Autodesk Inventor part; units mm, degrees
ref_plane "YZ Plane" through (0, 0, 0) normal (1, 0, 0) x (0, 1, 0)
ref_plane "XZ Plane" through (0, 0, 0) normal (0, 1, 0) x (-1, 0, 0)
ref_plane "XY Plane" through (0, 0, 0) normal (0, 0, 1) x (1, 0, 0)
sketch "Sketch1" plane through (0, 0, 0) normal (0, 1, 0) x (-1, 0, 0)
  line L0 (19, 32.5) -> (-11, 32.5)
  line L1 (-11, -32.5) -> (19, -32.5)
  line L2 (19, -32.5) -> (19, 32.5)
  line L3 (19, 32.5) -> (-19, -32.5) construction
  line L4 (-19, 32.5) -> (19, -32.5) construction
  line L5 (19, 19) -> (-19, 19) construction
  line L6 (-19, 19) -> (-19, -19) construction
  line L7 (-19, -19) -> (19, -19) construction
  line L8 (19, -19) -> (19, 19) construction
  line L9 (19, 19) -> (-19, -19) construction
  line L10 (-19, 19) -> (19, -19) construction
  line L11 (19, 32.5) -> (-11, 32.5) construction
  line L12 (-11, 32.5) -> (-11, -32.5) construction
  line L13 (-11, -32.5) -> (19, -32.5) construction
  line L14 (19, -32.5) -> (19, 32.5) construction
  line L15 (-21.9768, -11.3147) -> (-19, 12.5) construction
  line L16 (15.5, 29) -> (-7.5, 29) construction
  line L17 (-7.5, 29) -> (-7.5, -29) construction
  line L18 (-7.5, -29) -> (15.5, -29) construction
  line L19 (15.5, -29) -> (15.5, 29) construction
  line L20 (15, 15) -> (-15, 15) construction
  line L21 (-15, 15) -> (-15, -15) construction
  line L22 (-15, -15) -> (15, -15) construction
  line L23 (15, -15) -> (15, 15) construction
  line L24 (15, 15) -> (-15, -15) construction
  line L25 (-15, 15) -> (15, -15) construction
  circle A0 centre (15, 15) radius 1.25
  circle A1 centre (15, -15) radius 1.25
  circle A2 centre (-15, -15) radius 1.25
  circle A3 centre (-15, 15) radius 1.25
  circle A4 centre (-7.5, 29) radius 1.25
  circle A5 centre (15.5, 29) radius 1.25
  circle A6 centre (15.5, -29) radius 1.25
  circle A7 centre (-7.5, -29) radius 1.25
  circle A8 centre (0, 12) radius 2.5 construction
  circle A9 centre (0, -12) radius 2.5 construction
  line L26 (-4.75, 25.5) -> (-10.25, 25.5)
  line L27 (-10.25, 25.5) -> (-10.25, -25.5) construction
  line L28 (-10.25, -25.5) -> (-4.75, -25.5)
  line L29 (-4.75, -25.5) -> (-4.75, 25.5) construction
  line L30 (-4.75, 25.5) -> (-10.25, -25.5) construction
  line L31 (-10.25, 25.5) -> (-4.75, -25.5) construction
  line L32 (-11, 32.5) -> (-19, 32.5)
  line L33 (-19, 32.5) -> (-19, 19)
  line L34 (-19, -19) -> (-19, -32.5)
  line L35 (-19, -32.5) -> (-11, -32.5)
  arc A10 (-14.9077, -17.4983) -> (-15, -12.5) centre (-15, -15) ccw
  arc A11 (-15, 12.5) -> (-14.9077, 17.4983) centre (-15, 15) ccw
  line L36 (-15, 12.5) -> (-19, 12.5)
  line L37 (-19, 12.5) -> (-19, 19)
  line L38 (-15, -12.5) -> (-19, -12.5)
  line L39 (-19, -12.5) -> (-19, -19)
  line L40 (-14.9077, -17.4983) -> (-14.9077, -19)
  line L41 (-14.9077, 17.4983) -> (-14.9077, 19)
  arc A12 (15, 17.5) -> (15, 12.5) centre (15, 15) ccw
  line L42 (15, 12.5) -> (15, -12.5)
  line L43 (15, 17.5) -> (15, 19)
  line L44 (15, 19) -> (-4.75, 19)
  line L45 (-4.75, 19) -> (-4.75, 25.5)
  line L46 (-10.25, 25.5) -> (-10.25, 19)
  line L47 (-10.25, 19) -> (-14.9077, 19)
  line L48 (14.9077, -17.4983) -> (14.9077, -19)
  line L49 (14.9077, -19) -> (-4.75, -19)
  line L50 (-4.75, -19) -> (-4.75, -25.5)
  line L51 (-10.25, -25.5) -> (-10.25, -19)
  line L52 (-10.25, -19) -> (-14.9077, -19)
  arc A13 (15, -12.5) -> (14.9077, -17.4983) centre (15, -15) ccw
  point P0 (0, 0)
  point P1 (-7.5, 0)
  dimension "d0" = 38
  dimension "d2" = 38
  dimension "d3" = 38
  dimension "d4" = 30
  dimension "d8" = 65
  dimension "d9" = 23
  dimension "d10" = 58
  dimension "d11" = 3.5
  dimension "d13" = 3.5
  dimension "d14" = 2.5
  dimension "d15" = 2.5
  dimension "d16" = 2.5
  dimension "d17" = 2.5
  dimension "d18" = 2.5
  dimension "d19" = 2.5
  dimension "d20" = 2.5
  dimension "d21" = 2.5
  dimension "d22" = 5
  dimension "d23" = 5
  dimension "d24" = 7
  dimension "d25" = 7
  dimension "d31" = 5
  dimension "d32" = 5
  dimension "d33" = 4
  dimension "d34" = 5
  dimension "d36" = 5.5
  dimension "d37" = 51
extrude "Extrusion1" add sketch "Sketch1" along normal blind 4
fillet "Fillet1" radius 3 4 edges at (-19, 2, 32.5) (19, 2, 32.5) (19, 2, -32.5) (-19, 2, -32.5)
properties part number "coupler"
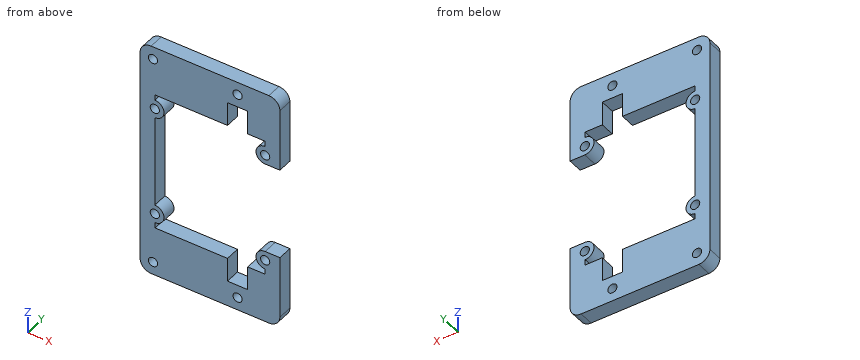
Verification items for the finished model (mm, model axes). Coordinates: 2 decimals unless noted, no trailing zeros. Order: outer loops, then holes, each group sorted by start corner. A loop starts at its lowest first (then second) coordinate and runs counter-clockwise, first axis right, second up.
Item 1: Section check D-D, the plane y = 3. Give the number of separate pieces and of enclosed holes in the cut face, then the cut area to 3 significant figures.
Filled in:
separate pieces: 1
enclosed holes: 8
area: 1,150 mm2
Item 2: Depth check by flat-ended pin: pin 1 (1 mm diameter, centred on y = 1, z = 11, fed in from +X); pin 2 (1.2 mm diameter, centred on x = 17.5, y = 2, fed in from +Z). Enter the tip coordinate at first touch or a pass-through.
Filled in:
pin 1: stops at x = -15
pin 2: stops at z = 32.36
Item 3: Section check A-A, the plane z = 15. Enter the section's corners in (x, y).
Filled in:
outline: (-19, 0) - (-16.25, 0) - (-16.25, 4) - (-19, 4) - close; (-13.75, 0) - (-12.5, 0) - (-12.5, 4) - (-13.75, 4) - close; (12.5, 0) - (13.75, 0) - (13.75, 4) - (12.5, 4) - close; (16.25, 0) - (19, 0) - (19, 4) - (16.25, 4) - close
Item 4: Section check C-C, the plane x = -2. Enter the section's corners in (y, z).
Filled in:
outline: (0, -32.5) - (4, -32.5) - (4, -19) - (0, -19) - close; (0, 19) - (4, 19) - (4, 32.5) - (0, 32.5) - close
Item 5: Material ranges on L1, parallel to Z at x = 7.5, y = 2.1; L2, parallel to Z at x = 11.5, y = 3.05; L3, parallel to Z at x = 7, y = 1.75, recorded low to high.
Filled in:
L1: z = -32.5 to -30.25, -27.75 to -25.5, 25.5 to 27.75, 30.25 to 32.5
L2: z = -32.5 to -19, 19 to 32.5
L3: z = -32.5 to -30.15, -27.85 to -25.5, 25.5 to 27.85, 30.15 to 32.5
Item 6: Section check B-B, the plane x = 7.5. Enter the section's corners in (y, z), then the cut area to 3 significant figures.
Filled in:
outline: (0, -32.5) - (4, -32.5) - (4, -30.25) - (0, -30.25) - close; (0, -27.75) - (4, -27.75) - (4, -25.5) - (0, -25.5) - close; (0, 25.5) - (4, 25.5) - (4, 27.75) - (0, 27.75) - close; (0, 30.25) - (4, 30.25) - (4, 32.5) - (0, 32.5) - close
area: 36.0 mm2
